from build123d import *

# Parameters (mm, degrees)
SKETCH6_R           = 3.687499751
CUT_EXTRUDE3_DEPTH  = 29.1338
SKETCH7_R           = 3.133725
BOSS_EXTRUDE1_DEPTH = 3.81
SKETCH8_R           = 2.159
BOSS_EXTRUDE2_DEPTH = 6.35
SKETCH9_R           = 4.699
CUT_EXTRUDE4_DEPTH  = 6.35
SKETCH10_W          = 6.35
SKETCH10_H          = 6.35
BOSS_EXTRUDE3_DEPTH = 3.81


with BuildPart() as part:
    # Sketch1 → Revolve1 (revolve)
    with BuildSketch(Plane(origin=(0, 0, 0), x_dir=(0, 0, -1), z_dir=(1, 0, 0))):
        Polygon((4.892085627, 0), (44.3738, 0), (44.3738, 2.159), (43.409235, 3.123565), (25.3238, 3.123565), (18.9738, 3.133725), (6.4516, 3.133725), (6.2738, 3.133725), (6.2738, 3.311525), (6.2738, 4.445), (6.2738, 4.699), (6.0198, 4.699), (0.635, 4.699), (0, 4.699), (0, 4.064), (0, 3.19405), (0, 0), align=None)
    revolve(axis=Axis((0, 0, -4.892085627), (0, 0, -1)))

    # Sketch6 → Cut-Extrude3 (cut)
    with BuildSketch(Plane(origin=(0, 0, -44.3738), x_dir=(-1, 0, 0), z_dir=(0, 0, -1))):
        Circle(SKETCH6_R)
    extrude(amount=-CUT_EXTRUDE3_DEPTH, mode=Mode.SUBTRACT)

    # Sketch7 → Boss-Extrude1 (add)
    with BuildSketch(Plane(origin=(0, 0, -15.24), x_dir=(-1, 0, 0), z_dir=(0, 0, -1))):
        Circle(SKETCH7_R)
    extrude(amount=BOSS_EXTRUDE1_DEPTH)

    # Sketch8 → Boss-Extrude2 (add)
    with BuildSketch(Plane(origin=(0, 0, -19.05), x_dir=(-1, 0, 0), z_dir=(0, 0, -1))):
        Circle(SKETCH8_R)
    extrude(amount=BOSS_EXTRUDE2_DEPTH)

    # Sketch9 → Cut-Extrude4 (cut)
    with BuildSketch(Plane.XY):
        Circle(SKETCH9_R)
    extrude(amount=-CUT_EXTRUDE4_DEPTH, mode=Mode.SUBTRACT)

    # Sketch10 → Boss-Extrude3 (add)
    with BuildSketch(Plane.XY.offset(-6.35)):
        Rectangle(SKETCH10_W, SKETCH10_H)
    extrude(amount=BOSS_EXTRUDE3_DEPTH)


solid = part.part
Input: part model. Units: mm. Frame: model coordinates. A direction names the side the tool comes from. Coordinates: 2 decimals unless noted, no trailing zeros. Loops run counter-clockwise (first coordinate to the right, second up) from the corner with the lowest first, then second, coordinate; pieces in that order, holes last.
Q1. Cut plane A-A (y = 0). Output: boundary loops of the cut face in (x, z) (3 decimals).
Q2. Contact query for flat-ended pins moving along their axis: pin 1 (1.5 mm diameter, centred on y = 1, z = -13, fed in from +X); pin 2 (1 mm diameter, centred on y = 1.5, z = -10.5, fed in from -X); pin 3 (3 mm diameter, centred on x = 2, z = -19.5, fed in from +Y). Output: stop coordinate, or through.
Q3. Cut plane C-C (z = -10). Output: boundary loops of the cut face in (x, y), then the cut area to 3 significant figures.
Q4. Material intervals for line 1 (Z direction, x = 2.5, y = 2.25); line 2 (X direction, y = 0, z = -19); line 3 (Z direction, x = -1.5, y = -1.75), sorted ascending.
Q5. Set-up query: faces 1 (the face through (0, 0, -2.54)), 2 (the face through (0.28, 2.14, -22.18)). Return all of +Z, -Z, +X, -X, +Y, -Y with unobstructed straight access to the full face (end or side cutting, diameter ignored); none if empty.
Working result:
1. outline: (-3.175, -6.35) - (-3.134, -6.35) - (-3.134, -19.05) - (-2.159, -19.05) - (-2.159, -25.4) - (2.159, -25.4) - (2.159, -19.05) - (3.134, -19.05) - (3.134, -6.35) - (3.175, -6.35) - (3.175, -2.54) - (-3.175, -2.54) - close
2. pin 1: stops at x = 3.12
2. pin 2: stops at x = -2.97
2. pin 3: stops at y = 3.08
3. outline: circle Ø6.27 at (0, 0)
3. area: 30.9 mm2
4. line 1: z = -6.35 to -2.54
4. line 2: x = -3.13 to 3.13
4. line 3: z = -19.05 to -2.54
5. face 1: +Z, +X, -X, +Y, -Y
5. face 2: -Z
